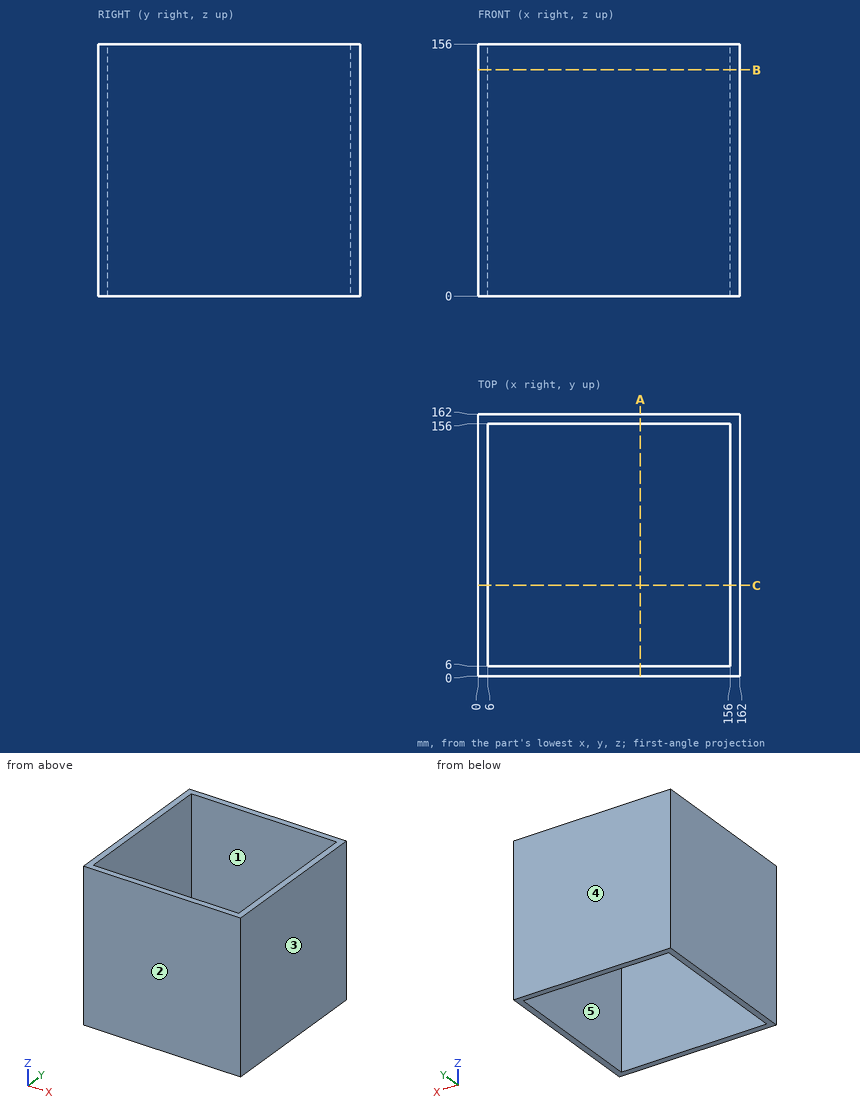
Input: dimensioned drawing with shaded views. Units: mm. Origin: part minimum x, y, z. A direction names the side the tool comes from. Coordinates: 2 decimals unless noted, no trailing zeros. Write each loop counter-clockwise with the first axis right and the second up, starting at its lowest first coordinate (ties: lowest second). Pieces come first, ordered by that corner, then holes. Notation, with made-up numbers: M 22,71 L 42,71 A15 ccw 42,93 Z; hole C 83.25,31 d7. An arc over 180 degrees is marked long. Answer as CSV lines item,"result". Start each with the question number.
Q1. Reachability of the marked faces 4 and 5 from +Z, -Z, +X, -X, +Y, -Y: full face, straight path, thin tool, end or side. Return the list, or none.
Q2. Line query: line 1 (Y direction, x = 134, z = 98.5). Output: solid intervals per line, ascending. Write a range as from..to.
Q3. Cut plane B-B on z = 140. Return the cut outline in (x, y), then the cut area to 3 significant figures.
Q4. Mould query, pull axis X, two halves, no side actions, for the marked faces 1, 2 and 3. Classes: released by +X, released by -X, zero draft, split by the parting line, or undercut.
Q5. Cut plane A-A on x = 100.5. Return the cut outline in (y, z).
Findings below:
1,face 4,"+Z, -Z, +X, -X, +Y"
1,face 5,"+Z, -Z"
2,line 1,"y = 0..6, 156..162"
3,outline,"M 0,0 L 162,0 L 162,162 L 0,162 Z; hole M 6,6 L 156,6 L 156,156 L 6,156 Z"
3,area,"3,740 mm2"
4,face 1,"undercut"
4,face 2,"zero draft"
4,face 3,"released by +X"
5,outline,"M 0,0 L 6,0 L 6,156 L 0,156 Z; M 156,0 L 162,0 L 162,156 L 156,156 Z"
